from build123d import *


with BuildPart() as part:
    # Szkic1 → Obrót1 (revolve)
    with BuildSketch(Plane.XY, mode=Mode.PRIVATE) as obr_t1_sk:
        Polygon((-28.72, 46.880116473), (-28.72, 36.880116473), (-24.697095519, -13.119883527), (-24.697095519, -23.119883527), (-37.355095289, -23.119883527), (-40, -8.119883527), (-40, 6.880116473), (-50, 6.880116473), (-50, 46.880116473), align=None)
    revolve(obr_t1_sk.sketch.rotate(Axis((0, 46.880116473, 0), (0, -1, 0)), 270), axis=Axis((0, 46.880116473, 0), (0, -1, 0)))


solid = part.part
Can you work these out from the model? Positions are in its coordinate system, mm. A direction names the side the tool comes from. Coordinates: 2 decimals unless noted, no trailing zeros. Loops run counter-clockwise (first coordinate to the right, second up) from the corner with the lowest first, then second, coordinate; pieces in that order, holes last. Notation, with made-up numbers: (16.5, -37.75) - (42.5, -37.75) arc R19 cw to (42.5, -4.75) - close; hole circle Ø2 at (14.25, -26). An arc over 180 degrees is marked (long way). Answer as a JSON object with one key per item and string values. Group by question number.
Item 1: On a 3-axis mill with a long thin cutter (end or side, diameter ignored), from which of +Z, -Z, +X, -X, +Y, -Y can I reach the whole of each face in a straight line? I mean faces 1 (the face through (-34, 6.88, 22)), 2 (the face through (24, -23.12, -8)). Say none if no direction works.
Item 2: If we section it at C-C (y = 16): List the corners of the cut face in (x, z) for me.
Item 3: If we section it at B-B (z = 0): List the corners of the cut face in (x, y) for me, plus the area to 3 significant figures.
Item 4: If we section it at A-A (x = 0): List the corners of the cut face in (y, z) for me, plus the area to 3 significant figures.
Item 5: If I drill on L1, parallel to X at y = 43.5, z = 0; L2, parallel to X at y = 33.5, z = -6; L3, parallel to Y at x = 27, z = -36, over which ranges is the centre line in solid material (lowest first)? Write a range as from..to.
Item 6: If we mould it in two halves opening along Z, with no side actions, what happens to faces 3 (the face through (22, 46.88, 22)), 4 (the face through (36.63, -22.18, -8.13)), 5 (the face through (17.48, 41.81, -22.79))? For each: released by +Z, released by -Z, zero draft, split by the parting line, or undercut.
Item 7: For pin 1 (1.5 mm diameter, centred on x = 7, y = -1.5, fed in from -Z); pin 2 (2 mm diameter, centred on x = -29, y = -10.5, fed in from -Z); pin 3 (8 mm diameter, centred on y = 6.5, z = 0, fed in from -X), each with a flat end and sliding along its axis, tell me the tip position at first contact or that it passes through.
Returned:
{
 "1": {"face 1": "-Y", "face 2": "+Z, -Z, +X, -X, -Y"},
 "2": {"outline": "circle Ø100 at (0, 0); hole circle Ø54.08 at (0, 0)"},
 "3": {"outline": "(-50, 6.88) - (-40, 6.88) - (-40, -8.12) - (-37.36, -23.12) - (-24.7, -23.12) - (-24.7, -13.12) - (-28.72, 36.88) - (-28.72, 46.88) - (-50, 46.88) - close; (24.7, -23.12) - (37.36, -23.12) - (40, -8.12) - (40, 6.88) - (50, 6.88) - (50, 46.88) - (28.72, 46.88) - (28.72, 36.88) - (24.7, -13.12) - close", "area": "2,620 mm²"},
 "4": {"outline": "(-23.12, -37.36) - (-8.12, -40) - (6.88, -40) - (6.88, -50) - (46.88, -50) - (46.88, -28.72) - (36.88, -28.72) - (-13.12, -24.7) - (-23.12, -24.7) - close; (-23.12, 24.7) - (-13.12, 24.7) - (36.88, 28.72) - (46.88, 28.72) - (46.88, 50) - (6.88, 50) - (6.88, 40) - (-8.12, 40) - (-23.12, 37.36) - close", "area": "2,620 mm²"},
 "5": {"L1": "x = -50..-28.72, 28.72..50", "L2": "x = -49.64..-27.81, 27.81..49.64", "L3": "y = 6.88..46.88"},
 "6": {"face 3": "zero draft", "face 4": "split by the parting line", "face 5": "undercut"},
 "7": {"pin 1": "stops at z = -39.51", "pin 2": "stops at z = -28.01", "pin 3": "stops at x = -50"}
}
